Part model, mm, in its own coordinate system. A direction names the side the tool comes from. Round coordinates to 2 decimals unless told otherwise and drop trailing zeros. Write each loop counter-clockwise with the first axis right and the second up, starting at its lowest first coordinate (ties: lowest second). Pieces come first, ordered by that corner, then holes.
from build123d import *

# Parameters (mm, degrees)
SKETCH_1_R          = 2
EXTRUDE_1_DEPTH     = 180
SKETCH_2_R          = 5
CUT_EXTRUDE_1_DEPTH = 180
SKETCH_3_W          = 11.661291253
SKETCH_3_H          = 5


with BuildPart() as part:
    # Sketch 1 → Extrude 1 (new body)
    with BuildSketch(Plane.XY):
        with BuildLine():
            Line((-24, 5), (-29.580398915, 5))
            ThreePointArc((-29.580398915, 5), (-25.980762114, 15), (-19.120326477, 23.117376915))
            Line((-19.120326477, 23.117376915), (-16.330127019, 18.284609691))
            ThreePointArc((-16.330127019, 18.284609691), (-9.5, 16.454482672), (-7.669872981, 23.284609691))
            Line((-7.669872981, 23.284609691), (-10.460072439, 28.117376915))
            ThreePointArc((-10.460072439, 28.117376915), (0, 30), (10.460072439, 28.117376915))
            Line((10.460072439, 28.117376915), (7.669872981, 23.284609691))
            ThreePointArc((7.669872981, 23.284609691), (9.5, 16.454482672), (16.330127019, 18.284609691))
            Line((16.330127019, 18.284609691), (19.120326477, 23.117376915))
            ThreePointArc((19.120326477, 23.117376915), (25.980762114, 15), (29.580398915, 5))
            Line((29.580398915, 5), (24, 5))
            ThreePointArc((24, 5), (19, 0), (24, -5))
            Line((24, -5), (29.580398915, -5))
            ThreePointArc((29.580398915, -5), (25.980762114, -15), (19.120326477, -23.117376915))
            Line((19.120326477, -23.117376915), (16.330127019, -18.284609691))
            ThreePointArc((16.330127019, -18.284609691), (9.5, -16.454482672), (7.669872981, -23.284609691))
            Line((7.669872981, -23.284609691), (10.460072439, -28.117376915))
            ThreePointArc((10.460072439, -28.117376915), (0, -30), (-10.460072439, -28.117376915))
            Line((-10.460072439, -28.117376915), (-7.669872981, -23.284609691))
            ThreePointArc((-7.669872981, -23.284609691), (-9.5, -16.454482672), (-16.330127019, -18.284609691))
            Line((-16.330127019, -18.284609691), (-19.120326477, -23.117376915))
            ThreePointArc((-19.120326477, -23.117376915), (-25.980762114, -15), (-29.580398915, -5))
            Line((-29.580398915, -5), (-24, -5))
            ThreePointArc((-24, -5), (-19, 0), (-24, 5))
        make_face()
        with Locations(Location((-10, 0, 0), (0, 0, 180))):
            Circle(SKETCH_1_R, mode=Mode.SUBTRACT)
        with Locations(Location((10, 0, 0), (0, 0, 180))):
            Circle(SKETCH_1_R, mode=Mode.SUBTRACT)
    extrude(amount=EXTRUDE_1_DEPTH)

    # Sketch 2 → Cut-Extrude 1 (cut)
    with BuildSketch(Plane(origin=(0, 0, 0), x_dir=(-1, 0, 0), z_dir=(0, 0, -1))):
        Circle(SKETCH_2_R)
    extrude(amount=-CUT_EXTRUDE_1_DEPTH, mode=Mode.SUBTRACT)

    # Sketch 3 → Cut-Revolve 1 (revolve, cut)
    with BuildSketch(Plane(origin=(0, 0, 0), x_dir=(1, 0, 0), z_dir=(0, 1, 0))):
        with Locations((-27.411044542, -57.5)):
            Rectangle(SKETCH_3_W, SKETCH_3_H)
    cut_revolve_1 = revolve(axis=Axis((0, 0, -56.149742432), (0, 0, 1)), mode=Mode.SUBTRACT)

    # Mirror 1: Cut-Revolve 1 across plane
    add(cut_revolve_1.mirror(Plane.XY.offset(90)), mode=Mode.SUBTRACT)


solid = part.part
Q1. Two-plate mould, pull along Z, no slides. Class faces 1 (the cylindrical face through (-25.906, -15.129, 89.58)), 2 (the cylindrical face through (0.1, 21.58, 122.54)): released by +Z, released by -Z, zero draft, split by the parting line, or undercut.
Q2. Tool access for faces 3 (the flat face through (9.045, -25.667, 27.115)), 4 (the flat face through (-17.706, -20.667, 152.115)), 5 (the flat face through (-17.74, 20.73, 152.12)): list every direction of +Z, -Z, +X, -X, +Y, -Y with a clear straight run to the whole face (end or side of a thin tool).
Q3. Saw through at D-D, the plane y = -8.5. Write the cut outline in (x, z).
Q4. Wall check: line 1 (Z direction, x = -19, y = -21.5); line 2 (Y direction, x = -10, z = 37); line 3 (X direction, y = -18.5, z = 137.5). Give the ranges that are in metal, low to high.
Q5. Saw through at A-A, the plane y = 0. Write the cut outline in (x, z), and give its area (3 significant figures).
Q6. Drop flat-ended pins along their axis: P1, Ø2, axis at y = 12.5, z = 137, coming from the -X side; P2, Ø6, axis at x = -27.5, z = 14.5, coming from the +Y side; P3, Ø1, axis at x = -10, z = 100, coming from the -Y side. Give the stop position or say it passes through.
Q7. Saw through at C-C, the plane z = 62. Write the cut outline in (x, y).
Q8. Saw through at B-B, the plane x = 0. Write the cut outline in (y, z).
Computed:
1. face 1: zero draft
1. face 2: undercut
2. face 3: +Z, -Z, +X
2. face 4: +Z, -Z, -Y
2. face 5: +Z, -Z, +Y
3. outline: (-28.77, 0) - (28.77, 0) - (28.77, 55) - (19.84, 55) - (19.84, 60) - (28.77, 60) - (28.77, 120) - (19.84, 120) - (19.84, 125) - (28.77, 125) - (28.77, 180) - (-28.77, 180) - (-28.77, 125) - (-19.84, 125) - (-19.84, 120) - (-28.77, 120) - (-28.77, 60) - (-19.84, 60) - (-19.84, 55) - (-28.77, 55) - close
4. line 1: z = 0 to 55, 60 to 120, 125 to 180
4. line 2: y = -28.28 to -27.32, -16.2 to -2, 2 to 16.2, 27.32 to 28.28
4. line 3: x = -23.62 to -16.45, -7.55 to 7.55, 16.45 to 23.62
5. outline: (-19, 0) - (-12, 0) - (-12, 180) - (-19, 180) - close; (-8, 0) - (-5, 0) - (-5, 180) - (-8, 180) - close; (5, 0) - (8, 0) - (8, 180) - (5, 180) - close; (12, 0) - (19, 0) - (19, 180) - (12, 180) - close
5. area: 3,600 mm2
6. P1: stops at x = -27.71
6. P2: stops at y = 17.31
6. P3: stops at y = -28.46
7. outline: (-29.58, -5) arc R30 ccw to (-19.12, -23.12) - (-16.33, -18.28) arc R5 cw to (-7.67, -23.28) - (-10.46, -28.12) arc R30 ccw to (10.46, -28.12) - (7.67, -23.28) arc R5 cw to (16.33, -18.28) - (19.12, -23.12) arc R30 ccw to (29.58, -5) - (24, -5) arc R5 cw to (24, 5) - (29.58, 5) arc R30 ccw to (19.12, 23.12) - (16.33, 18.28) arc R5 cw to (7.67, 23.28) - (10.46, 28.12) arc R30 ccw to (-10.46, 28.12) - (-7.67, 23.28) arc R5 cw to (-16.33, 18.28) - (-19.12, 23.12) arc R30 ccw to (-29.58, 5) - (-24, 5) arc R5 cw to (-24, -5) - close; hole circle Ø4 at (-10, 0); hole circle Ø10 at (0, 0); hole circle Ø4 at (10, 0)
8. outline: (-30, 0) - (-5, 0) - (-5, 180) - (-30, 180) - (-30, 125) - (-21.58, 125) - (-21.58, 120) - (-30, 120) - (-30, 60) - (-21.58, 60) - (-21.58, 55) - (-30, 55) - close; (5, 0) - (30, 0) - (30, 55) - (21.58, 55) - (21.58, 60) - (30, 60) - (30, 120) - (21.58, 120) - (21.58, 125) - (30, 125) - (30, 180) - (5, 180) - close
